from build123d import *

# Parameters (mm, degrees)
SKETCH1_R           = 2.84
BOSS_EXTRUDE1_DEPTH = 3
SKETCH2_R           = 1.079696648
BOSS_EXTRUDE2_DEPTH = 45
CUT_EXTRUDE1_DEPTH  = 1.4


with BuildPart() as part:
    # Sketch1 → Boss-Extrude1 (new body)
    with BuildSketch(Plane(origin=(0, 0, 0), x_dir=(1, 0, 0), z_dir=(0, 1, 0))):
        with Locations(Location((0, 0, 0), (0, 0, 270))):
            Circle(SKETCH1_R)
    extrude(amount=BOSS_EXTRUDE1_DEPTH)

    # Sketch2 → Boss-Extrude2 (add)
    with BuildSketch(Plane(origin=(0, 3, 0), x_dir=(1, 0, 0), z_dir=(0, 1, 0))):
        with Locations(Location((0, 0, 0), (0, 0, 90))):
            Circle(SKETCH2_R)
    extrude(amount=BOSS_EXTRUDE2_DEPTH)

    # Sketch3 → Cut-Extrude1 (cut)
    with BuildSketch(Plane.XZ):
        Polygon((1.65122177, 0), (0.825610885, 1.43), (-0.825610885, 1.43), (-1.65122177, 0), (-0.825610885, -1.43), (0.825610885, -1.43), align=None)
    extrude(amount=-CUT_EXTRUDE1_DEPTH, mode=Mode.SUBTRACT)


solid = part.part
Work out the finished part from the listing and answer in its coordinate system (mm). A direction names the side the tool comes from. Give positions to 0.01 mm unless a question says otherwise; leave off trailing zeros. Order: outer loops, then holes, each group sorted by start corner. A loop starts at its lowest first (then second) coordinate and runs counter-clockwise, first axis right, second up. Notation, with made-up numbers: (-28.5, 36) -> (25.5, 36) arc R11 cw to (25.5, 40) -> close; hole circle Ø1 at (-22.5, -8). An arc over 180 degrees is marked (long way). Answer as a JSON object with one key per item and string values. Group by question number.
1. The mould has two halves that part along Z. Classify faces 1 (the flat face through (0, 1, -1.43)), 2 (the flat face through (-1, 3, 1)), 3 (the cylindrical face through (-0.05, 25.18, 1.08)): released by +Z, released by -Z, zero draft, split by the parting line, or undercut.
2. Consider line 1 along Y through (x, z) = (1.3, -0.4); line 2 along Y through (x, z) = (-0.5, -0.7); line 3 along X through (y, z) = (8, 0.7). Determine where each line is inside the solid, lowest interval first. Write a range as [from, to].
3. Section B-B on y = 28.5 is taken. Determine the outline of the cut face in (x, z).
4. Flat-ended cylindrical pins translate along their axes: pin 1 Ø0.9 at (x, z) = (0, 0) entering from -Y; pin 2 Ø3 at (y, z) = (41.5, -2) entering from +X. Find the tip coordinate at first contact, or state that the pin passes through.
5. Section A-A on x = 0 is taken. Determine the outline of the cut face in (y, z).
6. A tool of negligible diameter and unlimited length cuts with its end or side. For faces 4 (the flat face through (0, 48, 0)), 5 (the flat face through (1.23, 0.69, -0.73)), from which of +Z, -Z, +X, -X, +Y, -Y can it reach the whole face along a straight path? Write none if from no direction.
Result sheet:
{
 "1": {"face 1": "undercut", "face 2": "zero draft", "face 3": "split by the parting line"},
 "2": {"line 1": "y = [1.4, 3]", "line 2": "y = [1.4, 48]", "line 3": "x = [-0.82, 0.82]"},
 "3": {"outline": "circle Ø2.16 at (0, 0)"},
 "4": {"pin 1": "stops at y = 1.4", "pin 2": "stops at x = 0.96"},
 "5": {"outline": "(0, -2.84) -> (3, -2.84) -> (3, -1.08) -> (48, -1.08) -> (48, 1.08) -> (3, 1.08) -> (3, 2.84) -> (0, 2.84) -> (0, 1.43) -> (1.4, 1.43) -> (1.4, -1.43) -> (0, -1.43) -> close"},
 "6": {"face 4": "+Z, -Z, +X, -X, +Y", "face 5": "-Y"}
}
